Design review of the part built by this model. Coordinates are the model's own, in mm. A direction names the side the tool comes from. Coordinates: 2 decimals unless noted, no trailing zeros. Loops run counter-clockwise (first coordinate to the right, second up) from the corner with the lowest first, then second, coordinate; pieces in that order, holes last.
from build123d import *

# Parameters (mm, degrees)
F0_R          = 5
F0_W          = 20
F0_H          = 20
F1_DEPTH      = 10
F1_DEPTH_BACK = 10
F2_R          = 1.7
F3_DEPTH      = 25


with BuildPart() as f1:
    # F0 (on Front) → F1 (new body, two sides)
    with BuildSketch(Plane.XZ) as f1_sk:
        Polygon((10, -15), (150, -15), (150, 15), (-150, 15), (-150, -15), (-10, -15), (-10, 5), (10, 5), align=None)
        with Locations((-140, 0)):
            Circle(F0_R, mode=Mode.SUBTRACT)
        with Locations((140, 0)):
            Circle(F0_R, mode=Mode.SUBTRACT)
        Polygon((10, -35), (10, -15), (-10, -15), (-10, -35), (-1.5, -35), (-1.5, -29), (1.5, -29), (1.5, -35), align=None)
        with Locations((0, -5)):
            Rectangle(F0_W, F0_H)
    extrude(amount=F1_DEPTH)
    extrude(f1_sk.sketch, amount=-F1_DEPTH_BACK)

    # F2 (on face) → F3 (cut)
    with BuildSketch(Plane.YZ.offset(10)):
        with Locations((-6, -32)):
            Circle(F2_R)
        with Locations((6, -32)):
            Circle(F2_R)
    extrude(amount=-F3_DEPTH, mode=Mode.SUBTRACT)


solid = f1.part
Q1. Machinability: for faces 4 (the flat face through (150, 0, 0)), 5 (the flat face through (10, 0, -25)), 6 (the flat face through (-81, 0, -15)), 7 (the flat face through (-1.5, 0, -32)), which of the approach directions +Z, -Z, +X, -X, +Y, -Y give a long, thin tool a straight path to every point of the face, cutting with its end or side? Answer none if there is none.
Q2. The part is to be moulded in two halves that separate along X. For faces 1 (the flat face through (2, 0, 15)), 2 (the flat face through (-150, 0, 0)), 3 (the flat face through (1.5, 0, -32)), say which applies: pulls with the +X half, pulls with the -X half, needs draft (parallel to the pull), parting line crosses it, or undercut.
Q3. Take a section at D-D, the plane x = -66.5. Write out the cut boundary in (y, z), then the cut area to 3 significant figures.
Q4. Take a section at A-A, the plane z = 0. Write out the cut boundary in (x, y).
Q5. Take a section at C-C, the plane z = -22.5. Write out the cut boundary in (x, y).
Q6. Clearance check with flat-ended pins moving along their axes: pin 1 Ø2 at (y, z) = (-6, -32) entering from +X; pin 2 Ø1.5 at (x, y) = (117, -3.5) entering from -Z; pin 3 Ø10 at (y, z) = (0, -21.5) entering from +X; pin 4 Ø5 at (y, z) = (-4.5, -32) entering from -X. State where each tip first meets the part, or that it passes through.
Q7. For line 1 (X direction, y = -8.75, z = -3.5); line 2 (Z direction, x = 140, y = 4.5); line 3 (Z direction, x = -5, y = -6), list the stretches that pass through material, from the lowest coordinate up.
Q8. Take a section at B-B, the plane x = 140. Write out the cut boundary in (y, z).
Entries:
1. face 4: +Z, -Z, +X, +Y, -Y
1. face 5: -Z, +X, +Y, -Y
1. face 6: -Z, -X, +Y, -Y
1. face 7: -Z, +Y, -Y
2. face 1: needs draft
2. face 2: pulls with the -X half
2. face 3: undercut
3. outline: (-10, -15) - (10, -15) - (10, 15) - (-10, 15) - close
3. area: 600 mm2
4. outline: (-150, -10) - (-145, -10) - (-145, 10) - (-150, 10) - close; (-135, -10) - (135, -10) - (135, 10) - (-135, 10) - close; (145, -10) - (150, -10) - (150, 10) - (145, 10) - close
5. outline: (-10, -10) - (10, -10) - (10, 10) - (-10, 10) - close
6. pin 1: passes through
6. pin 2: stops at z = -15
6. pin 3: stops at x = 10
6. pin 4: stops at x = -10
7. line 1: x = -150 to -143.57, -136.43 to 136.43, 143.57 to 150
7. line 2: z = -15 to -5, 5 to 15
7. line 3: z = -35 to -33.7, -30.3 to 15
8. outline: (-10, -15) - (10, -15) - (10, -5) - (-10, -5) - close; (-10, 5) - (10, 5) - (10, 15) - (-10, 15) - close
